from build123d import *

# Parameters (mm, degrees)
SKETCH1_W                  = 200
SKETCH1_H                  = 83.89
WHEEL_STEERING_DUMMY_DEPTH = 340.92
MOUNT_BODY_DEPTH           = 10
MOUNT_BODY_DEPTH_BACK      = 10
SKETCH3_W                  = 20
SKETCH3_H                  = 30
SKETCH3_W_2                = 14
SKETCH3_H_2                = 24
MOUNT_TONGUE_DEPTH         = 35
SKETCH4_R                  = 5
MOUNT_BOLT_HOLES_DEPTH     = 359.639177203
FILLET1_R                  = 7.5


with BuildPart() as part:
    # Sketch1 → Wheel & Steering Dummy (new body)
    with BuildSketch(Plane(origin=(0, 0, 0), x_dir=(1, 0, 0), z_dir=(0, 1, 0))):
        Rectangle(SKETCH1_W, SKETCH1_H)
    extrude(amount=-WHEEL_STEERING_DUMMY_DEPTH)

    # Sketch2 → Mount Body (add, two sides: drawn at the far end of the back side and taken through both)
    with BuildSketch(Plane.XY.offset(-MOUNT_BODY_DEPTH_BACK)):
        Polygon((-15, 0), (15, 0), (15, 30), (60, 30), (60, 60), (15, 60), (-15, 60), align=None)
    extrude(amount=MOUNT_BODY_DEPTH + MOUNT_BODY_DEPTH_BACK)

    # Sketch3 → Mount Tongue (cut)
    with BuildSketch(Plane(origin=(60, 0, 0), x_dir=(0, 0, -1), z_dir=(1, 0, 0))):
        with Locations((0, 45)):
            Rectangle(SKETCH3_W, SKETCH3_H)
        with Locations((0, 45)):
            Rectangle(SKETCH3_W_2, SKETCH3_H_2, mode=Mode.SUBTRACT)
    extrude(amount=-MOUNT_TONGUE_DEPTH, mode=Mode.SUBTRACT)

    # Sketch4 → Mount Bolt Holes (cut, through all)
    with BuildSketch(Plane.XY.offset(7)):
        with Locations((35, 45)):
            Circle(SKETCH4_R)
        with Locations((50, 45)):
            Circle(SKETCH4_R)
    extrude(amount=-MOUNT_BOLT_HOLES_DEPTH, mode=Mode.SUBTRACT)

    # Fillet1
    fillet1_edges = [part.edges().sort_by_distance(p)[0] for p in [
        (-15, 60, 0),
        (15, 30, 0),
    ]]
    fillet(fillet1_edges, radius=FILLET1_R)


solid = part.part
Can you work these out from the model? Positions are in its coordinate system, mm. A direction names the side the tool comes from. Round coordinates to 2 decimals unless told otherwise and drop trailing zeros. Order: outer loops, then holes, each group sorted by start corner. A loop starts at its lowest first (then second) coordinate and runs counter-clockwise, first axis right, second up. Notation, with made-up numbers: (46.25, 27.5) -> (105.25, 27.5) arc R17 cw to (105.25, 59.5) -> close; hole circle Ø11 at (35, 52.5). An arc over 180 degrees is marked (long way). Write each question's results on one line, items separated by ' | '. Start each with the question number.
Item 1: Which directions (+Z, -Z, +X, -X, +Y, -Y) give clear straight access to the entire face, cutting with the end or side of a thin tool? Please do faces 5 (the flat face through (43, 57, 0)), 6 (the flat face through (-15, 27, 0)), 7 (the flat face through (5, 30, -10)), 8 (the flat face through (15, 11, 0)), 9 (the flat face through (43, 45, -7)).
Item 2: If we section it at B-B, the plane y = 45: Write out the boundary of the cut face in (x, z).
Item 3: Will these pins go through, and if not, where does the flat tip stop? pin 1 (12 mm diameter, centred on x = 12.5, y = 40.5, fed in from -Z); pin 2 (1 mm diameter, centred on x = 26.5, z = -22.5, fed in from +Y); pin 3 (12 mm diameter, centred on x = -24, y = 11, fed in from +Z); pin 4 (6 mm diameter, centred on y = 29.5, z = -0.5, fed in from -X).
Item 4: Please list where these lines run through material, in increasing order: L1, parallel to Y at x = 35, z = -1; L2, parallel to Y at x = -82.5, z = -3; L3, parallel to Y at x = 21, z = -2.5.
Item 5: If we section it at C-C, the plane x = 1.5: Write out the boundary of the cut face in (y, z) (3 decimals), then the cut area to 3 significant figures.
Item 6: Thinking about a two-plate mould opening in Y: for faces 1 (the flat face through (43, 33, 0)), 2 (the flat face through (-1, -340.92, -1)), 3 (the flat face through (5, 30, 10)), 4 (the flat face through (9, 60, 0)), which applies, +Y half, -Y half, draft (parallel to the pull), parting line (faces both ways), or undercut?
Item 7: If we section it at A-A, the plane x = 35: Write out the boundary of the cut face in (y, z) (3 decimals).
Item 8: If we section it at D-D, the plane z = 14: Write out the boundary of the cut face in (x, y).
Results:
1) face 5: +Z, -Z, +X, +Y | face 6: +Z, -Z, -X, +Y | face 7: -Z, +X, -X, +Y | face 8: +Z, -Z, +X | face 9: -Z, +X, +Y
2) outline: (-15, -10) -> (25, -10) -> (25, -7) -> (30, -7) -> (30, 7) -> (25, 7) -> (25, 10) -> (-15, 10) -> close; (40, -7) -> (45, -7) -> (45, 7) -> (40, 7) -> close; (55, -7) -> (60, -7) -> (60, 7) -> (55, 7) -> close
3) pin 1: stops at z = -10 | pin 2: stops at y = 0 | pin 3: passes through | pin 4: stops at x = -15
4) L1: y = -340.92 to 0, 33 to 40, 50 to 57 | L2: y = -340.92 to 0 | L3: y = -340.92 to 0, 29.85 to 60
5) outline: (-340.92, -41.945) -> (0, -41.945) -> (0, -10) -> (60, -10) -> (60, 10) -> (0, 10) -> (0, 41.945) -> (-340.92, 41.945) -> close | area: 29,800 mm2
6) face 1: undercut | face 2: -Y half | face 3: draft | face 4: +Y half
7) outline: (-340.92, -41.945) -> (0, -41.945) -> (0, 41.945) -> (-340.92, 41.945) -> close; (33, -7) -> (40, -7) -> (40, 7) -> (33, 7) -> close; (50, -7) -> (57, -7) -> (57, 7) -> (50, 7) -> close
8) outline: (-100, -340.92) -> (100, -340.92) -> (100, 0) -> (-100, 0) -> close
